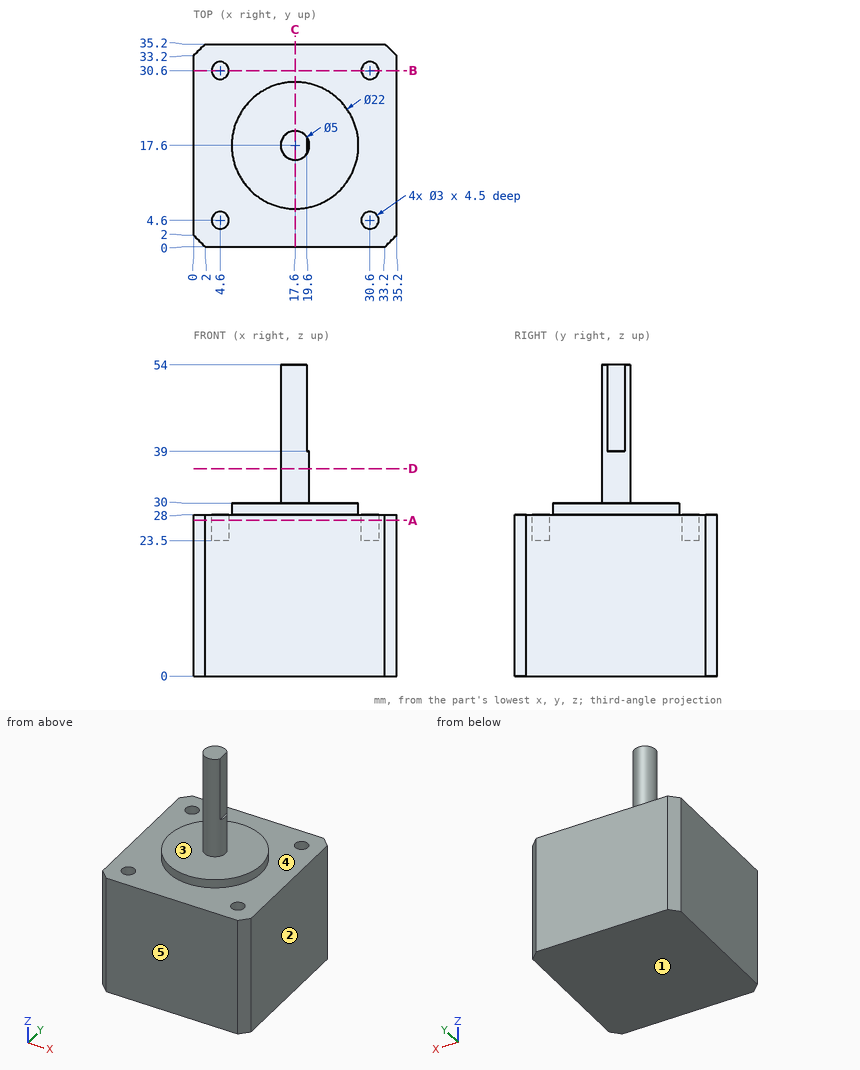
Print and shaded views of the part. All mm, measured from the part's lowest x, y and z. A direction names the side the tool comes from. Round coordinates to 2 decimals unless told otherwise and drop trailing zeros. Order: outer loops, then holes, each group sorted by start corner. A loop starts at its lowest first (then second) coordinate and runs counter-clockwise, first axis right, second up. Notation, with made-up numbers: (41.25, 8) - (95.25, 8) arc R17 ccw to (95.25, 34) - close; hole circle Ø6 at (-39, 41). An arc over 180 degrees is marked (long way). Use a Markdown table: item, result.
1) Wall check: L1, parallel to Y at x = 4.6, z = 24.7; L2, parallel to X at y = 30, z = 26. Give the ranges that are in metal, low to high.
Recorded:
| item | result |
|---|---|
| L1 | y = 0 to 3.1, 6.1 to 29.1, 32.1 to 35.2 |
| L2 | x = 0 to 3.23, 5.97 to 29.23, 31.97 to 35.2 |
2) Saw through at D-D on z = 36. Write the cut outline in (x, y).
Recorded:
| item | result |
|---|---|
| outline | circle Ø5 at (17.6, 17.6) |
3) Tool access for the marked faces 4 and 5: list every direction of +Z, -Z, +X, -X, +Y, -Y with a clear straight run to the whole face (end or side of a thin tool).
Recorded:
| item | result |
|---|---|
| face 4 | +Z |
| face 5 | +Z, -Z, +X, -X, -Y |
4) Pull direction Z, two halves, no side cores. Call the marked faces 1, 2 and 3: pulls with the +Z half, pulls with the -Z half, needs draft (parallel to the pull), parting line crosses it, or undercut.
Recorded:
| item | result |
|---|---|
| face 1 | pulls with the -Z half |
| face 2 | needs draft |
| face 3 | pulls with the +Z half |
5) Saw through at B-B on y = 30.6. Write the cut outline in (x, z), and give its area (3 significant figures).
Recorded:
| item | result |
|---|---|
| outline | (0, 0) - (35.2, 0) - (35.2, 28) - (32.1, 28) - (32.1, 23.5) - (29.1, 23.5) - (29.1, 28) - (6.1, 28) - (6.1, 23.5) - (3.1, 23.5) - (3.1, 28) - (0, 28) - close |
| area | 959 mm² |
6) Saw through at C-C on x = 17.6. Write the cut outline in (y, z), and give its area (3 significant figures).
Recorded:
| item | result |
|---|---|
| outline | (0, 0) - (35.2, 0) - (35.2, 28) - (28.6, 28) - (28.6, 30) - (20.1, 30) - (20.1, 54) - (15.1, 54) - (15.1, 30) - (6.6, 30) - (6.6, 28) - (0, 28) - close |
| area | 1,150 mm² |
7) Flat gauge pins, fed straight in: pin 1 Ø1.8 at (x, y) = (30.6, 4.6) entering from -Z; pin 2 Ø1.5 at (x, y) = (30, 30) entering from +Z; pin 3 Ø1.5 at (x, y) = (4.5, 31) entering from +Z; pin 4 Ø12 at (x, y) = (6.5, 25.5) entering from +Z. Where does each tip first touch, or does it go through?
Recorded:
| item | result |
|---|---|
| pin 1 | stops at z = 0 |
| pin 2 | stops at z = 28 |
| pin 3 | stops at z = 23.5 |
| pin 4 | stops at z = 30 |
8) Saw through at A-A on z = 27. Write the cut outline in (x, y), and give its area (3 significant figures).
Recorded:
| item | result |
|---|---|
| outline | (0, 2) - (2, 0) - (33.2, 0) - (35.2, 2) - (35.2, 33.2) - (33.2, 35.2) - (2, 35.2) - (0, 33.2) - close; hole circle Ø3 at (4.6, 4.6); hole circle Ø3 at (4.6, 30.6); hole circle Ø3 at (30.6, 4.6); hole circle Ø3 at (30.6, 30.6) |
| area | 1,200 mm² |
